For this review, take the finished solid that the model builds, in its own axes (mm). A direction names the side the tool comes from. Round coordinates to 2 decimals unless told otherwise and drop trailing zeros. Loops run counter-clockwise (first coordinate to the right, second up) from the corner with the lowest first, then second, coordinate; pieces in that order, holes last.
1. Tool access review of faces 4 (the cylindrical face through (200.485, 29.452, 3.757)), 5 (the flat face through (77.57, -7.76, 3.86)): name each direction out of +Z, -Z, +X, -X, +Y, -Y from which nothing blocks a thin tool from reaching the whole face with its end or side.
2. To check wall thickness, follow line 1 along Y through (x, z) = (102, 6.75); line 2 along Y through (x, z) = (88, 3.25); line 3 along Y through (x, z) = (139, 4.5). State the ranges of each line that lie inside material, in increasing order.
3. Draft analysis for pull direction Y (two halves, no side actions). For faces 1 (the cylindrical face through (284.876, -76.888, 3.757)), 2 (the flat face through (252.45, -27.31, 3.76)), 3 (the flat face through (253.79, -41.225, 3.863)), state which applies: released by +Y, released by -Y, zero draft, split by the parting line, or undercut.
4. Clearance check with flat-ended pins moving along their axes: pin 1 Ø2 at (y, z) = (-75.5, 5.5) entering from +X; pin 2 Ø4 at (x, y) = (214.98, -62.84) entering from +Z; pin 3 Ø2 at (x, z) = (35.5, 4.5) entering from -Y; pin 4 Ø2 at (x, z) = (85.5, 6.5) entering from +Y. State where each tip first meets the part, or that it passes through.
5. Consider section B-B on z = 3.75. State how many separate pieces and enclosed holes the cut face has, then the cut area to 3 significant figures.
6. Consider section A-A on x = -24. State the section outline as (y, z) points.
7. Consider section C-C on x = 57.5. State the section outline as (y, z) points.
from build123d import *

# Parameters (mm, degrees)
SKETCH1_R               = 27.4955
SKETCH1_R_2             = 3.29946
SKETCH1_R_3             = 9.525
SKETCH1_R_4             = 52.4256
BOSS_EXTRUDE1_DEPTH     = 7.62
CUT_EXTRUDE1_DEPTH      = 314.319493614
CUT_EXTRUDE1_DEPTH_BACK = 314.319493614
SKETCH2_R               = 4.49961
SKETCH2_R_2             = 2.50063
CUT_EXTRUDE2_DEPTH      = 314.319493614
CUT_EXTRUDE2_DEPTH_BACK = 314.319493614


with BuildPart() as part:
    # Sketch1 → Boss-Extrude1 (new body)
    # profile 1 of 5: a face of its own
    with BuildSketch(Plane.XY):
        with BuildLine():
            ThreePointArc((57.285987503, -118.460322704), (55.688968414, -123.739787041), (51.433442898, -127.248877555))
            Line((51.433442898, -127.248877555), (276.360987503, -82.143687357))
            ThreePointArc((276.360987503, -82.143687357), (267.780420135, -68.483534561), (283.811267218, -66.684131167))
            Line((283.811267218, -66.684131167), (220.199398147, 13.174615234))
            ThreePointArc((220.199398147, 13.174615234), (230.216497711, -4.968011872), (233.68508, -25.4))
            ThreePointArc((233.68508, -25.4), (126.817436716, -67.969857276), (175.144631834, 36.420602736))
            Line((175.144631834, 36.420602736), (5.000495975, 45.701244141))
            ThreePointArc((5.000495975, 45.701244141), (34.230844848, 30.689704088), (45.974, 0))
            ThreePointArc((45.974, 0), (15.172060928, -43.398355305), (-35.960016757, -28.644124543))
            Line((-35.960016757, -28.644124543), (40.310707788, -124.394878894))
            ThreePointArc((40.310707788, -124.394878894), (44.617604714, -109.468950749), (57.285987503, -118.460322704))
        make_face()
    # profile 2 of 5: a face of its own
    with BuildSketch(Plane.XY):
        with BuildLine():
            ThreePointArc((0, 45.974), (-41.415538495, 19.959004162), (-35.960016757, -28.644124543))
            ThreePointArc((-35.960016757, -28.644124543), (15.172060928, -43.398355305), (45.974, 0))
            ThreePointArc((45.974, 0), (34.230844848, 30.689704088), (5.000495975, 45.701244141))
            Line((5.000495975, 45.701244141), (0, 45.974))
        make_face()
        with Locations(Location((0, 0, 0), (0, 0, 180))):
            Circle(SKETCH1_R, mode=Mode.SUBTRACT)
    # profile 3 of 5: a face of its own
    with BuildSketch(Plane.XY):
        with BuildLine():
            ThreePointArc((40.310707788, -124.394878894), (43.625834707, -127.040890072), (47.760987503, -127.985322704))
            Line((47.760987503, -127.985322704), (51.433442898, -127.248877555))
            ThreePointArc((51.433442898, -127.248877555), (55.688968414, -123.739787041), (57.285987503, -118.460322704))
            ThreePointArc((57.285987503, -118.460322704), (44.617604714, -109.468950749), (40.310707788, -124.394878894))
        make_face()
        with Locations(Location((47.760987503, -118.460322704, 0), (0, 0, 180))):
            Circle(SKETCH1_R_2, mode=Mode.SUBTRACT)
    # profile 4 of 5: a face of its own
    with BuildSketch(Plane.XY):
        with Locations((276.360987503, -72.618687357)):
            Circle(SKETCH1_R_3)
        with Locations(Location((276.360987503, -72.618687357, 0), (0, 0, 180))):
            Circle(SKETCH1_R_2, mode=Mode.SUBTRACT)
    # profile 5 of 5: a face of its own
    with BuildSketch(Plane.XY):
        with BuildLine():
            ThreePointArc((233.68508, -25.4), (230.216497711, -4.968011872), (220.199398147, 13.174615234))
            ThreePointArc((220.199398147, 13.174615234), (200.160512587, 29.620750083), (175.144631834, 36.420602736))
            ThreePointArc((175.144631834, 36.420602736), (126.817436716, -67.969857276), (233.68508, -25.4))
        make_face()
        with Locations(Location((171.77258, -25.4, 0), (0, 0, 180))):
            Circle(SKETCH1_R_4, mode=Mode.SUBTRACT)
    extrude(amount=BOSS_EXTRUDE1_DEPTH)

    # Sketch2 → Cut-Extrude1 (cut, two sides: drawn at the far end of the back side and taken through both)
    with BuildSketch(Plane.XY.offset(7.62).offset(-CUT_EXTRUDE1_DEPTH_BACK)):
        with Locations((0, 38.354)):
            Circle(SKETCH2_R)
        with Locations((171.77258, 31.76905)):
            Circle(SKETCH2_R_2)
        with Locations((24.653475982, 29.380868571)):
            Circle(SKETCH2_R)
        with Locations((37.771316559, 6.660102206)):
            Circle(SKETCH2_R)
        with Locations((33.215538337, -19.177)):
            Circle(SKETCH2_R)
        with Locations((13.117840577, -36.040970778)):
            Circle(SKETCH2_R)
        with Locations((-13.117840577, -36.040970778)):
            Circle(SKETCH2_R)
        with Locations((-33.215538337, -19.177)):
            Circle(SKETCH2_R)
        with Locations((-37.771316559, 6.660102206)):
            Circle(SKETCH2_R)
        with Locations((-24.653475982, 29.380868571)):
            Circle(SKETCH2_R)
        with Locations((202.680501925, 22.693665281)):
            Circle(SKETCH2_R_2)
        with Locations((223.775377024, -1.651118351)):
            Circle(SKETCH2_R_2)
        with Locations((228.359731502, -33.536004105)):
            Circle(SKETCH2_R_2)
        with Locations((214.978065204, -62.837766042)):
            Circle(SKETCH2_R_2)
        with Locations((187.878962629, -80.253301783)):
            Circle(SKETCH2_R_2)
        with Locations((155.666197371, -80.253301783)):
            Circle(SKETCH2_R_2)
        with Locations((128.567094796, -62.837766042)):
            Circle(SKETCH2_R_2)
        with Locations((115.185428498, -33.536004105)):
            Circle(SKETCH2_R_2)
        with Locations((119.769782976, -1.651118351)):
            Circle(SKETCH2_R_2)
        with Locations((140.864658075, 22.693665281)):
            Circle(SKETCH2_R_2)
    extrude(amount=CUT_EXTRUDE1_DEPTH + CUT_EXTRUDE1_DEPTH_BACK, mode=Mode.SUBTRACT)

    # Sketch5 → Cut-Extrude2 (cut, two sides: drawn at the far end of the back side and taken through both)
    with BuildSketch(Plane(origin=(0, 0, 0), x_dir=(-1, 0, 0), z_dir=(0, 0, -1)).offset(-CUT_EXTRUDE2_DEPTH_BACK)):
        with BuildLine():
            Line((-265.98852685, -56.539497078), (-241.245162788, -25.476519923))
            ThreePointArc((-241.245162788, -25.476519923), (-238.464669174, -24.646277907), (-236.720158772, -26.965141853))
            ThreePointArc((-236.720158772, -26.965141853), (-227.620878985, -59.228125128), (-204.753887162, -83.739299465))
            ThreePointArc((-204.753887162, -83.739299465), (-203.801270663, -86.826655842), (-206.649906438, -88.351294098))
            Line((-206.649906438, -88.351294098), (-258.038190746, -78.04629414))
            ThreePointArc((-258.038190746, -78.04629414), (-259.622077281, -77.008967427), (-260.048409115, -75.164249445))
            ThreePointArc((-260.048409115, -75.164249445), (-260.880500131, -66.879818937), (-265.649679181, -60.054930991))
            ThreePointArc((-265.649679181, -60.054930991), (-266.530067918, -58.365742929), (-265.98852685, -56.539497078))
        make_face()
        with BuildLine():
            Line((-131.754965097, 31.155997891), (-38.12708703, 36.26300177))
            ThreePointArc((-38.12708703, 36.26300177), (-35.701196113, 34.830725487), (-36.08930912, 32.040433318))
            ThreePointArc((-36.08930912, 32.040433318), (-45.105625086, 17.161299066), (-48.259972129, 0.05186645))
            ThreePointArc((-48.259972129, 0.05186645), (-48.840291996, -1.561342946), (-50.313400987, -2.438363815))
            Line((-50.313400987, -2.438363815), (-105.593039761, -13.227704597))
            ThreePointArc((-105.593039761, -13.227704597), (-107.469894435, -12.860469717), (-108.558589456, -11.288150386))
            ThreePointArc((-108.558589456, -11.288150386), (-117.439212577, 9.856745234), (-133.131943584, 26.581286223))
            ThreePointArc((-133.131943584, 26.581286223), (-134.048834262, 29.351858), (-131.754965097, 31.155997891))
        make_face()
        with BuildLine():
            Line((-172.497020686, -95.200043594), (-66.759785208, -116.403752218))
            ThreePointArc((-66.759785208, -116.403752218), (-64.898408853, -116.057311266), (-63.793790983, -114.519597825))
            ThreePointArc((-63.793790983, -114.519597825), (-53.348385706, -102.924522715), (-37.910600393, -105.210795401))
            ThreePointArc((-37.910600393, -105.210795401), (-36.067318036, -105.691160666), (-34.408414964, -104.754954902))
            Line((-34.408414964, -104.754954902), (7.552696475, -52.076707806))
            ThreePointArc((7.552696475, -52.076707806), (7.7901592, -49.267572092), (5.287657457, -47.969451515))
            ThreePointArc((5.287657457, -47.969451515), (-23.30510003, -42.259909046), (-43.390999871, -21.124600118))
            ThreePointArc((-43.390999871, -21.124600118), (-44.541450027, -19.963260096), (-46.161306381, -19.743461099))
            Line((-46.161306381, -19.743461099), (-105.477050266, -31.320558719))
            ThreePointArc((-105.477050266, -31.320558719), (-106.846053421, -32.079030552), (-107.510559814, -33.496027522))
            ThreePointArc((-107.510559814, -33.496027522), (-129.012430096, -74.048972037), (-171.989119852, -90.16963803))
            ThreePointArc((-171.989119852, -90.16963803), (-174.524763167, -92.454466996), (-172.497020686, -95.200043594))
        make_face()
    extrude(amount=CUT_EXTRUDE2_DEPTH + CUT_EXTRUDE2_DEPTH_BACK, mode=Mode.SUBTRACT)


solid = part.part
Resolved:
1. face 4: +Z, -Z, +X, +Y
1. face 5: +Z, -Z
2. line 1: y = -117.11 to -109.34, -30.64 to -12.53, 32.78 to 40.41
2. line 2: y = -119.92 to -112.14, -27.91 to -9.79, 33.54 to 41.17
2. line 3: y = -109.69 to -101.92, -81.27 to -66.32, 15.52 to 21.03, 24.36 to 38.39
3. face 1: split by the parting line
3. face 2: released by +Y
3. face 3: undercut
4. pin 1: stops at x = 285.7
4. pin 2: passes through
4. pin 3: stops at y = -119.61
4. pin 4: stops at y = 41.36
5. separate pieces: 1
5. enclosed holes: 27
5. area: 14,200 mm2
6. outline: (-43.66, 0) - (-13.42, 0) - (-13.42, 7.62) - (-43.66, 7.62) - close; (13.42, 0) - (24.93, 0) - (24.93, 7.62) - (13.42, 7.62) - close; (33.83, 0) - (39.21, 0) - (39.21, 7.62) - (33.83, 7.62) - close
7. outline: (-126.03, 0) - (-105.13, 0) - (-105.13, 7.62) - (-126.03, 7.62) - close; (-21.96, 0) - (-3.84, 0) - (-3.84, 7.62) - (-21.96, 7.62) - close; (35.21, 0) - (42.84, 0) - (42.84, 7.62) - (35.21, 7.62) - close
